from build123d import *

# Parameters (mm, degrees)
REVOLVE_1_ANGLE = 180
SKETCH_2_W      = 10
SKETCH_2_H      = 10
EXTRUDE_1_DEPTH = 200
SKETCH_5_W      = 10
SKETCH_5_H      = 10
EXTRUDE_3_DEPTH = 200
SKETCH_6_W      = 10
SKETCH_6_H      = 10
EXTRUDE_4_DEPTH = 200


with BuildPart() as part:
    # ｽｹｯﾁ1 → 回転1 (revolve)
    with BuildSketch(Plane.XY):
        with BuildLine():
            Line((0, 70), (0, 150))
            ThreePointArc((0, 150), (-150, 0), (0, -150))
            Line((0, -150), (0, -70))
            ThreePointArc((0, -70), (-70, 0), (0, 70))
        make_face()
    revolve(axis=Axis((0, 150, 0), (0, -1, 0)), revolution_arc=REVOLVE_1_ANGLE)

    # ｽｹｯﾁ2 → ﾎﾞｽ - 押し出し1 (add)
    with BuildSketch(Plane(origin=(0, 0, 0), x_dir=(1, 0, 0), z_dir=(0, 1, 0))):
        with Locations((0, 120)):
            Rectangle(SKETCH_2_W, SKETCH_2_H)
    extrude(amount=EXTRUDE_1_DEPTH)

    # ｽｹｯﾁ5 → ﾎﾞｽ - 押し出し3 (add)
    with BuildSketch(Plane(origin=(0, 0, 0), x_dir=(0, 0, -1), z_dir=(0.8660254037844364, -0.5000000000000041, 0))):
        with Locations((120, 0)):
            Rectangle(SKETCH_5_W, SKETCH_5_H)
    extrude(amount=EXTRUDE_3_DEPTH)

    # ｽｹｯﾁ6 → ﾎﾞｽ - 押し出し4 (add)
    with BuildSketch(Plane(origin=(0, 0, 0), x_dir=(0, 0, -1), z_dir=(-0.8660254037844434, -0.49999999999999206, 0))):
        with Locations((120, 0)):
            Rectangle(SKETCH_6_W, SKETCH_6_H)
    extrude(amount=EXTRUDE_4_DEPTH)


solid = part.part
Part model, mm, in its own coordinate system. A direction names the side the tool comes from. Coordinates: 2 decimals unless noted, no trailing zeros. Order: outer loops, then holes, each group sorted by start corner. A loop starts at its lowest first (then second) coordinate and runs counter-clockwise, first axis right, second up. Notation, with made-up numbers: M 80,39.5 L 97,39.5 A26 ccw 97,72.5 Z; hole C 3.25,-9.75 d11. An arc over 180 degrees is marked long. Use a Markdown table: item, result.
(1) Cut at B-B on y = -84.5. Write the cut outline in (x, z), then the cut area to 3 significant figures.
A:
| item | result |
|---|---|
| outline | M -156.36,-125 L -136.36,-125 L -136.36,-115 L -156.36,-115 Z; M -123.93,0 A123.93 ccw 123.93,0 Z; M 136.36,-125 L 156.36,-125 L 156.36,-115 L 136.36,-115 Z |
| area | 24,500 mm^2 |
(2) Cut at D-D on x = 51. Write the cut outline in (y, z).
A:
| item | result |
|---|---|
| outline | M -141.06,0 A141.06 ccw 141.06,0 L 47.95,0 A47.95 cw -47.95,0 Z |
(3) Flat gauge pins, fed straight in: pin 1 (4 mm diameter, centred on x = -14.5, y = 88, fed in from -Z); pin 2 (8 mm diameter, centred on x = -0.5, y = 150, fed in from +Z); pin 3 (4 mm diameter, centred on x = -58.5, z = -82, fed in from +Y); pin 4 (10 mm diameter, centred on x = 135, y = -71, fed in from -Z). Where does each tip first touch, or does it go through?
A:
| item | result |
|---|---|
| pin 1 | stops at z = -122.06 |
| pin 2 | stops at z = 0 |
| pin 3 | stops at y = 112.93 |
| pin 4 | stops at z = -125 |
(4) Cut at C-C on z = -55. Write the cut outline in (x, y).
A:
| item | result |
|---|---|
| outline | C 0,0 d279.11; hole C 0,0 d86.6 |
(5) Tool access for faces 1 (the flat face through (-5, 141, -120)), 2 (the flat face through (128, -74, -115)), 3 (the flat face through (0, 147, -115)): list every direction of +Z, -Z, +X, -X, +Y, -Y with a clear straight run to the whole face (end or side of a thin tool).
A:
| item | result |
|---|---|
| face 1 | -Z, -X, +Y |
| face 2 | +X, -Y |
| face 3 | +X, -X, +Y |
(6) Pull direction X, two halves, no side cores. Call faces 4 (the flat face through (124.23, -65.95, -119.93)), 5 (the flat face through (119.23, -74.61, -119.93)), 6 (the flat face through (31, -65, 0)): released by +X, released by -X, zero draft, split by the parting line, or undercut.
A:
| item | result |
|---|---|
| face 4 | released by +X |
| face 5 | undercut |
| face 6 | zero draft |
(7) Cut at A-A on x = -98.5. Write the cut outline in (y, z).
A:
| item | result |
|---|---|
| outline | M -113.13,0 A113.13 ccw 113.13,0 Z; M -62.64,-125 L -51.1,-125 L -51.1,-115 L -62.64,-115 Z |
(8) Probe L1, parallel to X at y = 17, z = -39.5; L2, parallel to Y at x = -38.5, z = -11; L3, parallel to X at y = 181.5, z = -118.5. List the from-to ranges inside material, lowest first.
A:
| item | result |
|---|---|
| L1 | x = -143.7 to -55.23, 55.23 to 143.7 |
| L2 | y = -144.56 to -57.42, 57.42 to 144.56 |
| L3 | x = -5 to 5 |
